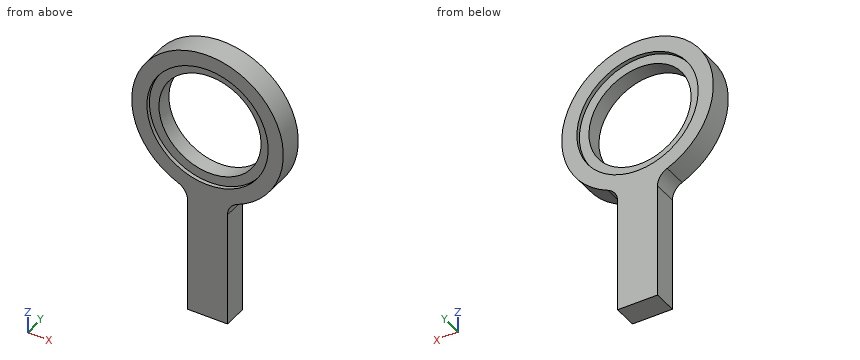
from build123d import *

# Parameters (mm, degrees)
SKETCH_1_R      = 9.5
SKETCH_1_R_2    = 6.4
EXTRUDE_1_DEPTH = 2
SKETCH_2_R      = 9.5
SKETCH_2_R_2    = 7.6
EXTRUDE_2_DEPTH = 0.5
EXTRUDE_START   = -2.5
SKETCH_2_2_R    = 9.5
SKETCH_2_2_R_2  = 7.6
EXTRUDE_3_DEPTH = 0.5
EXTRUDE_START_2 = -3
EXTRUDE_4_DEPTH = 3
FILLET_1_R      = 2


with BuildPart() as part:
    # 草图1 → 凸台-拉伸1 (new body)
    with BuildSketch(Plane(origin=(0, 0, 0), x_dir=(1, 0, 0), z_dir=(0, 1, 0))):
        with Locations(Location((0, 0, 0), (0, 0, 270))):
            Circle(SKETCH_1_R)
        with Locations(Location((0, 0, 0), (0, 0, 270))):
            Circle(SKETCH_1_R_2, mode=Mode.SUBTRACT)
    extrude(amount=EXTRUDE_1_DEPTH)

    # 草图2 → 凸台-拉伸2 (add)
    with BuildSketch(Plane(origin=(0, 2, 0), x_dir=(1, 0, 0), z_dir=(0, 1, 0))):
        with Locations(Location((0, 0, 0), (0, 0, 270))):
            Circle(SKETCH_2_R)
        with Locations(Location((0, 0, 0), (0, 0, 270))):
            Circle(SKETCH_2_R_2, mode=Mode.SUBTRACT)
    extrude(amount=EXTRUDE_2_DEPTH)

    # 草图2<2> → 凸台-拉伸3 (add)
    with BuildSketch(Plane(origin=(0, 2, 0), x_dir=(1, 0, 0), z_dir=(0, 1, 0)).offset(EXTRUDE_START)):
        with Locations(Location((0, 0, 0), (0, 0, 270))):
            Circle(SKETCH_2_2_R)
        with Locations(Location((0, 0, 0), (0, 0, 270))):
            Circle(SKETCH_2_2_R_2, mode=Mode.SUBTRACT)
    extrude(amount=EXTRUDE_3_DEPTH)

    # 草图4 → 凸台-拉伸4 (add)
    with BuildSketch(Plane(origin=(0, 2.5, 0), x_dir=(1, 0, 0), z_dir=(0, 1, 0)).offset(EXTRUDE_START_2)):
        with BuildLine():
            Line((-2.5, 25), (-2.5, 9.16515139))
            ThreePointArc((-2.5, 9.16515139), (0, 9.5), (2.5, 9.16515139))
            Line((2.5, 9.16515139), (2.5, 25))
            Line((2.5, 25), (-2.5, 25))
        make_face()
    extrude(amount=EXTRUDE_4_DEPTH)

    # 圆角1
    fillet_1_edges = [part.edges().sort_by_distance(p)[0] for p in [
        (2.5, 1, -9.16515139),
        (-2.5, 1, -9.16515139),
    ]]
    fillet(fillet_1_edges, radius=FILLET_1_R)


solid = part.part
The listing builds one solid part. Answer for the finished solid, in the listing's coordinates (mm). Give positions to 0.01 mm unless a question says otherwise; leave off trailing zeros. Order: outer loops, then holes, each group sorted by start corner. A loop starts at its lowest first (then second) coordinate and runs counter-clockwise, first axis right, second up. Notation, with made-up numbers: (33, 88.25) - (84, 88.25) arc R12 ccw to (84, 110.25) - close; hole circle Ø1 at (-20, -30.5). An arc over 180 degrees is marked (long way). One line per item, written item: value. Start each with the question number.
1) A cutting plane is placed at B-B on z = 0. Give the vertices of the cut face in (x, y).
2) A cutting plane is placed at A-A on x = 0. Give the vertices of the cut face in (y, z).
3) Find the intervals of material crossed by L1, parallel to X at y = -0.05, z = 0; L2, parallel to Y at x = -2.5, z = -6; L3, parallel to Z at x = 5.5, y = 0.7, in increasing order.
4) A cutting plane is placed at C-C on y = 0.45. Give the vertices of the cut face in (x, z).
5) Given pin 1 Ø10 at (x, z) = (0, 0) entering from +Y; pin 2 Ø7.5 at (x, z) = (2.5, 1.5) entering from +Y; pin 3 Ø0.9 at (y, z) = (1.5, -19.5) entering from +X, each flat-ended and moving along its own axis, determine where each tip first touches the part or whether it passes through.
Answer sheet:
1. outline: (-9.5, -0.5) - (-7.6, -0.5) - (-7.6, 0) - (-6.4, 0) - (-6.4, 2) - (-7.6, 2) - (-7.6, 2.5) - (-9.5, 2.5) - close; (6.4, 0) - (7.6, 0) - (7.6, -0.5) - (9.5, -0.5) - (9.5, 2.5) - (7.6, 2.5) - (7.6, 2) - (6.4, 2) - close
2. outline: (-0.5, -25) - (2.5, -25) - (2.5, -7.6) - (2, -7.6) - (2, -6.4) - (0, -6.4) - (0, -7.6) - (-0.5, -7.6) - close; (-0.5, 7.6) - (0, 7.6) - (0, 6.4) - (2, 6.4) - (2, 7.6) - (2.5, 7.6) - (2.5, 9.5) - (-0.5, 9.5) - close
3. L1: x = -9.5 to -7.6, 7.6 to 9.5
3. L2: y = 0 to 2
3. L3: z = -7.75 to -3.27, 3.27 to 7.75
4. outline: (-3.72, -8.74) arc R2 cw to (-2.5, -10.58) - (-2.5, -25) - (2.5, -25) - (2.5, -10.58) arc R2 cw to (3.72, -8.74) arc R9.5 ccw (long way) to start; hole circle Ø12.8 at (0, 0)
5. pin 1: passes through
5. pin 2: stops at y = 2
5. pin 3: stops at x = 2.5
